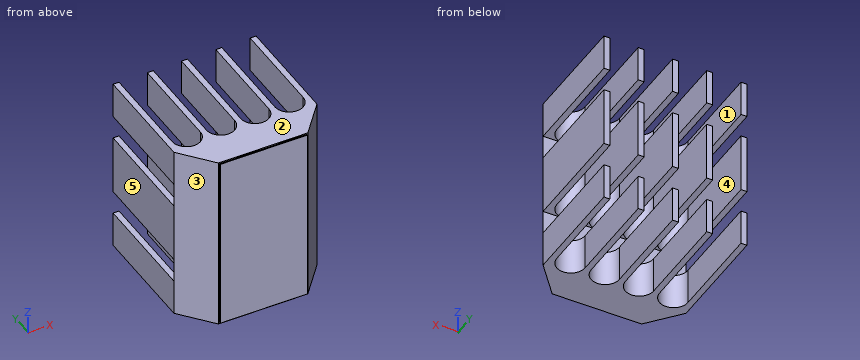
from build123d import *

# Parameters (mm, degrees)
AUFSATZ_LINEAR_AUSTRAGEN1_DEPTH = 7.5
SCHNITT_LINEAR_AUSTRAGEN1_DEPTH = 15
SCHNITT_LINEAR_AUSTRAGEN2_REACH = 20.554
SKIZZE3_W                       = 2
SKIZZE3_H                       = 9.3
SKIZZE4_W                       = 7.3
SKIZZE4_H                       = 14.8
AUFSATZ_LINEAR_AUSTRAGEN2_DEPTH = 0.1


with BuildPart() as part:
    # Skizze1 → Aufsatz-Linear austragen1 (new, symmetric)
    with BuildSketch(Plane.XY):
        Polygon((-6, 12), (-6, 2.7), (-3.75, 0), (3.75, 0), (6, 2.7), (6, 12), align=None)
    extrude(amount=AUFSATZ_LINEAR_AUSTRAGEN1_DEPTH, both=True)

    # Skizze2 → Schnitt-Linear austragen1 (cut)
    with BuildSketch(Plane.XY.offset(7.5)):
        with BuildLine():
            Line((-3.125, 12), (-3.125, 3.8875))
            ThreePointArc((-3.125, 3.8875), (-4.3125, 2.7), (-5.5, 3.8875))
            Line((-5.5, 3.8875), (-5.5, 12))
            ThreePointArc((-5.5, 12), (-4.3125, 13.1875), (-3.125, 12))
        make_face()
        with BuildLine():
            Line((-0.25, 12), (-0.25, 3.8875))
            ThreePointArc((-0.25, 3.8875), (-1.4375, 2.7), (-2.625, 3.8875))
            Line((-2.625, 3.8875), (-2.625, 12))
            ThreePointArc((-2.625, 12), (-1.4375, 13.1875), (-0.25, 12))
        make_face()
        with BuildLine():
            Line((2.625, 12), (2.625, 3.8875))
            ThreePointArc((2.625, 3.8875), (1.4375, 2.7), (0.25, 3.8875))
            Line((0.25, 3.8875), (0.25, 12))
            ThreePointArc((0.25, 12), (1.4375, 13.1875), (2.625, 12))
        make_face()
        with BuildLine():
            Line((5.5, 12), (5.5, 3.8875))
            ThreePointArc((5.5, 3.8875), (4.3125, 2.7), (3.125, 3.8875))
            Line((3.125, 3.8875), (3.125, 12))
            ThreePointArc((3.125, 12), (4.3125, 13.1875), (5.5, 12))
        make_face()
    extrude(amount=-SCHNITT_LINEAR_AUSTRAGEN1_DEPTH, mode=Mode.SUBTRACT)

    # Schnitt-Linear austragen2: up to this face of the body (flat: up to its plane)
    schnitt_linear_austragen2_end = Plane(part.part.faces().sort_by_distance((-6, 7.35, 0))[0])
    # Skizze3 → Schnitt-Linear austragen2 (cut, up to the picked face)
    with BuildSketch(Plane(origin=(6, 0, 0), x_dir=(0, 0, -1), z_dir=(1, 0, 0)), mode=Mode.PRIVATE) as schnitt_linear_austragen2_sk1:
        with Locations((-3.5, 7.35)):
            Rectangle(SKIZZE3_W, SKIZZE3_H)
    schnitt_linear_austragen2_tool1 = split(extrude(schnitt_linear_austragen2_sk1.sketch, amount=-SCHNITT_LINEAR_AUSTRAGEN2_REACH, mode=Mode.PRIVATE), bisect_by=schnitt_linear_austragen2_end, keep=Keep.BOTH, mode=Mode.PRIVATE)
    # Skizze3 → Schnitt-Linear austragen2 (cut, up to the picked face)
    with BuildSketch(Plane(origin=(6, 0, 0), x_dir=(0, 0, -1), z_dir=(1, 0, 0)), mode=Mode.PRIVATE) as schnitt_linear_austragen2_sk2:
        with Locations((3.5, 7.35)):
            Rectangle(SKIZZE3_W, SKIZZE3_H)
    schnitt_linear_austragen2_tool2 = split(extrude(schnitt_linear_austragen2_sk2.sketch, amount=-SCHNITT_LINEAR_AUSTRAGEN2_REACH, mode=Mode.PRIVATE), bisect_by=schnitt_linear_austragen2_end, keep=Keep.BOTH, mode=Mode.PRIVATE)
    # Skizze3 → Schnitt-Linear austragen2 (cut, up to the picked face)
    with BuildSketch(Plane(origin=(6, 0, 0), x_dir=(0, 0, -1), z_dir=(1, 0, 0)), mode=Mode.PRIVATE) as schnitt_linear_austragen2_sk3:
        with Locations((10.5, 7.35)):
            Rectangle(SKIZZE3_W, SKIZZE3_H)
    schnitt_linear_austragen2_tool3 = split(extrude(schnitt_linear_austragen2_sk3.sketch, amount=-SCHNITT_LINEAR_AUSTRAGEN2_REACH, mode=Mode.PRIVATE), bisect_by=schnitt_linear_austragen2_end, keep=Keep.BOTH, mode=Mode.PRIVATE)
    # Skizze3 → Schnitt-Linear austragen2 (cut, up to the picked face)
    with BuildSketch(Plane(origin=(6, 0, 0), x_dir=(0, 0, -1), z_dir=(1, 0, 0)), mode=Mode.PRIVATE) as schnitt_linear_austragen2_sk4:
        with Locations((17.5, 7.35)):
            Rectangle(SKIZZE3_W, SKIZZE3_H)
    schnitt_linear_austragen2_tool4 = split(extrude(schnitt_linear_austragen2_sk4.sketch, amount=-SCHNITT_LINEAR_AUSTRAGEN2_REACH, mode=Mode.PRIVATE), bisect_by=schnitt_linear_austragen2_end, keep=Keep.BOTH, mode=Mode.PRIVATE)
    add(schnitt_linear_austragen2_tool1.solids().sort_by(Axis((6, 7.35, 3.5), (-1, 0, 0)))[0], mode=Mode.SUBTRACT)
    add(schnitt_linear_austragen2_tool2.solids().sort_by(Axis((6, 7.35, -3.5), (-1, 0, 0)))[0], mode=Mode.SUBTRACT)
    add(schnitt_linear_austragen2_tool3.solids().sort_by(Axis((6, 7.35, -10.5), (-1, 0, 0)))[0], mode=Mode.SUBTRACT)
    add(schnitt_linear_austragen2_tool4.solids().sort_by(Axis((6, 7.35, -17.5), (-1, 0, 0)))[0], mode=Mode.SUBTRACT)

    # Skizze4 → Aufsatz-Linear austragen2 (add)
    with BuildSketch(Plane.XZ):
        Rectangle(SKIZZE4_W, SKIZZE4_H)
    extrude(amount=AUFSATZ_LINEAR_AUSTRAGEN2_DEPTH)


solid = part.part
CAD build for the part. Positions are in the model's coordinates, mm. Face numbers are marked on the shaded views. A direction names the side the tool comes from. Round coordinates to 2 decimals unless told otherwise and drop trailing zeros. Write each loop counter-clockwise with the first axis right and the second up, starting at its lowest first coordinate (ties: lowest second). Pieces come first, ordered by that corner, then holes.
(1) 3-axis set-ups, long thin cutter, end or side, ignore diameter. For the marked faces 4 and 5: which of +Z, -Z, +X, -X, +Y, -Y reach the whole face in a straight line?
(2) Mould opens along X. For the marked faces 1, 2 and 3 say: pulls with the +X half, pulls with the -X half, needs draft (parallel to the pull), parting line crosses it, or undercut.
(3) Probe line 1 along X through (y, z) = (7, 1) (3 decimals); line 2 along Y through (x, z) = (-1, 2.75); line 3 along Y through (x, z) = (-0.75, -5). List the from-to ranges inside material, lowest first.
(4) Slice it at B-B, the plane x = 0. Write the cut outline in (y, z), and give its area (3 significant figures).
(5) Slice it at D-D, the plane z = -3.5. Write the cut outline in (x, y), and give its area (3 significant figures).
(6) Drop flat-ended pins along their axis: P1, Ø0.6, axis at x = 1, z = -3.5, coming from the +Y side; P2, Ø1.5, axis at x = -4.5, z = -1.5, coming from the +Y side. Give the stop position or say it passes through.
(7) Slice it at C-C, the plane y = 7.5. Count the separate pieces of the cut face and the enclosed holes in it, and give its area (3 significant figures).
From the geometry:
1. face 4: +Z, -Z, +Y
1. face 5: +Z, -Z, -X, +Y, -Y
2. face 1: undercut
2. face 2: needs draft
2. face 3: pulls with the -X half
3. line 1: x = -6 to -5.5, -3.125 to -2.625, -0.25 to 0.25, 2.625 to 3.125, 5.5 to 6
3. line 2: y = -0.1 to 2.7
3. line 3: y = -0.1 to 2.92
4. outline: (-0.1, -7.4) - (0, -7.4) - (0, -7.5) - (12, -7.5) - (12, -4.5) - (2.7, -4.5) - (2.7, -2.5) - (12, -2.5) - (12, 2.5) - (2.7, 2.5) - (2.7, 4.5) - (12, 4.5) - (12, 7.5) - (0, 7.5) - (0, 7.4) - (-0.1, 7.4) - close
4. area: 144 mm2
5. outline: (-6, 2.7) - (-3.75, 0) - (-3.65, 0) - (-3.65, -0.1) - (3.65, -0.1) - (3.65, 0) - (3.75, 0) - (6, 2.7) - close
5. area: 27.1 mm2
6. P1: stops at y = 2.7
6. P2: stops at y = 3.16
7. separate pieces: 15
7. enclosed holes: 0
7. area: 27.5 mm2
